Check sheet for the drawn part. Datum: minimum x, y, z corner. Units: mm. A direction names the side the tool comes from. Coordinates: 2 decimals unless noted, no trailing zeros. Write each loop counter-clockwise with the first axis right and the second up, starting at its lowest first coordinate (ties: lowest second). Pieces come first, ordered by that corner, then holes. Notation, with made-up numbers: (52.25, -23) -> (66.25, -23) arc R13 ccw to (66.25, -10) -> close; hole circle Ø4 at (79.5, 72.5). An arc over 180 degrees is marked (long way). One line per question, with ' | ' between items.
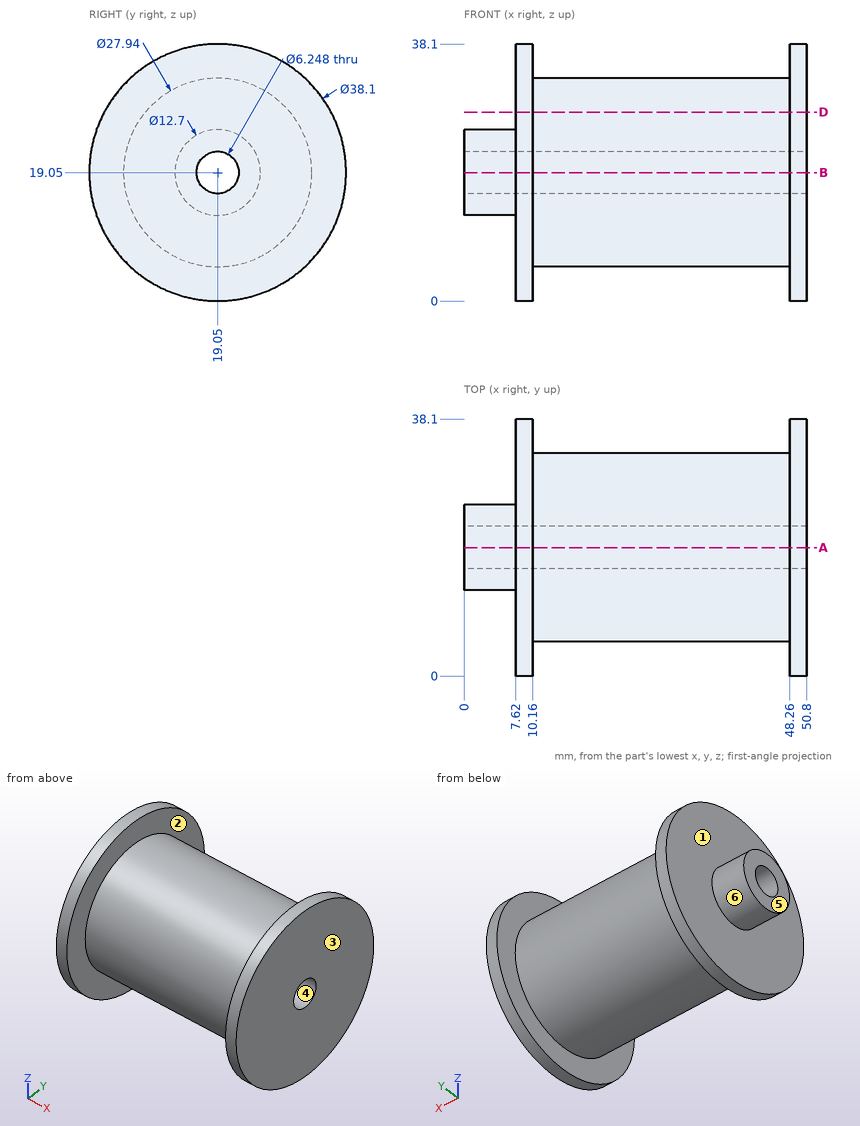
1. Cross-section at A-A on y = 19.05. Record the boundary of the cut face in (x, z) (1 decimal), and give its area (3 significant figures).
Worked answers:
outline: (0, 12.7) -> (7.6, 12.7) -> (7.6, 0) -> (10.2, 0) -> (10.2, 5.1) -> (48.3, 5.1) -> (48.3, 0) -> (50.8, 0) -> (50.8, 15.9) -> (0, 15.9) -> close; (0, 22.2) -> (50.8, 22.2) -> (50.8, 38.1) -> (48.3, 38.1) -> (48.3, 33) -> (10.2, 33) -> (10.2, 38.1) -> (7.6, 38.1) -> (7.6, 25.4) -> (0, 25.4) -> close | area: 1,040 mm²
2. Cross-section at D-D on z = 28. Record the boundary of the cut face in (x, y), and give its area (3 significant figures).
Worked answers:
outline: (7.62, 2.23) -> (10.16, 2.23) -> (10.16, 8.32) -> (48.26, 8.32) -> (48.26, 2.23) -> (50.8, 2.23) -> (50.8, 35.87) -> (48.26, 35.87) -> (48.26, 29.78) -> (10.16, 29.78) -> (10.16, 35.87) -> (7.62, 35.87) -> close | area: 988 mm²
3. Material ranges on line 1 (X direction, y = 29.5, z = 9.5); line 2 (Y direction, x = 12, z = 19), recorded low to high. Write a range as from..to.
Worked answers:
line 1: 7.62..10.16, 48.26..50.8 | line 2: 5.08..15.93, 22.17..33.02
4. Go/stop test with flat-tipped pins: P1, Ø10, axis at x = 34, y = 20, coming from the +Z side; P2, Ø8, axis at x = 33.5, y = 33.5, coming from the -Z side; P3, Ø1, axis at x = 6, y = 22.5, coming from the -Z side. Record where each tip stops, or that it passes through.
Worked answers:
P1: z = 33.02 | P2: z = 9.78 | P3: z = 13.43
5. Tool access check on the marked faces 1, 2 and 3. Record the directions out of +Z, -Z, +X, -X, +Y, -Y that give a thin tool (end or side, any length) a straight path to the whole face; none if there is none.
Worked answers:
face 1: -X | face 2: none | face 3: +Z, -Z, +X, +Y, -Y
6. Mould release check, pull along Y, two halves, no side actions. Record for the marked faces 4, 5 and 6: released by +Y, released by -Y, zero draft, split by the parting line, or undercut.
Worked answers:
face 4: undercut | face 5: zero draft | face 6: split by the parting line
